from build123d import *

# Parameters (mm, degrees)
EXTRUDE_1_DEPTH     = 95
CUT_EXTRUDE_1_REACH = 144.466
SKETCH_2_R          = 3


with BuildPart() as part:
    # 草图1 → 凸台-拉伸1 (new body)
    with BuildSketch(Plane.XY):
        Polygon((-43.550332336, 35.659057411), (-38.550332336, 35.659057411), (-38.550332336, -8.806832193), (56.449667664, -8.806832193), (56.449667664, -14.340942589), (-43.550332336, -14.340942589), align=None)
    extrude(amount=EXTRUDE_1_DEPTH)

    # 草图2 → 切除-拉伸1 (cut, up to next)
    with BuildSketch(Plane.ZY.offset(43.550332336), mode=Mode.PRIVATE) as cut_extrude_1_sk1:
        with Locations((27, 8.8)):
            Circle(SKETCH_2_R)
    cut_extrude_1_tool1 = extrude(cut_extrude_1_sk1.sketch, amount=-CUT_EXTRUDE_1_REACH, mode=Mode.PRIVATE) & part.part
    add(cut_extrude_1_tool1.solids().sort_by_distance((-43.550332, 8.8, 27))[0], mode=Mode.SUBTRACT)


solid = part.part
Geometry: final body of the model. Coordinates: model frame, mm. A direction names the side the tool comes from. Round coordinates to 2 decimals unless told otherwise and drop trailing zeros. Loops run counter-clockwise (first coordinate to the right, second up) from the corner with the lowest first, then second, coordinate; pieces in that order, holes last. Notation, with made-up numbers: M 23.5,-37.75 L 81.5,-37.75 A17 ccw 81.5,-20.75 Z; hole C 61,23 d7. An arc over 180 degrees is marked long. Put each result on its own line as item: value. Start each with the question number.
(1) Section query C-C (z = 57). Return loops of the section in (x, y), then the cut area to 3 significant figures.
(2) Material intervals for line 1 along Y through (x, z) = (-40, 27); line 2 along X through (y, z) = (10, 88); line 3 along Y through (x, z) = (16, 49.5), sorted ascending. Write a range as [from, to].
(3) Draft query along Z for faces 3 (the face through (-4, -10, 0)), 4 (the face through (-41.1, 8.9, 24)), 5 (the face through (8, -8.807, 47)). Return one class per face: +Z half, -Z half, draft (parallel to the pull), parting line (faces both ways), or undercut.
(4) Section query A-A (y = 8.8). Return loops of the section in (x, z).
(5) Contact query for flat-ended pins moving along their axis: pin 1 Ø3 at (y, z) = (24.5, 34) entering from +X; pin 2 Ø10 at (x, z) = (-33, 85) entering from +Y. Output: stop coordinate, or through.
(6) Set-up query: faces 1 (the face through (56.45, -12, 47)), 2 (the face through (-38.55, 14, 47)). Return all of +Z, -Z, +X, -X, +Y, -Y with unobstructed straight access to the full face (end or side cutting, diameter ignored); none if empty.
(7) Section query D-D (y = 18). Return loops of the section in (x, z).
(8) Section query B-B (z = 27). Return loops of the section in (x, y), then the cut area to 3 significant figures.
Findings below:
1. outline: M -43.55,-14.34 L 56.45,-14.34 L 56.45,-8.81 L -38.55,-8.81 L -38.55,35.66 L -43.55,35.66 Z
1. area: 776 mm2
2. line 1: y = [-14.34, 5.8], [11.8, 35.66]
2. line 2: x = [-43.55, -38.55]
2. line 3: y = [-14.34, -8.81]
3. face 3: -Z half
3. face 4: undercut
3. face 5: draft
4. outline: M -43.55,0 L -38.55,0 L -38.55,24 L -43.55,24 Z; M -43.55,30 L -38.55,30 L -38.55,95 L -43.55,95 Z
5. pin 1: stops at x = -38.55
5. pin 2: stops at y = -8.81
6. face 1: +Z, -Z, +X, +Y, -Y
6. face 2: +Z, -Z, +X, +Y
7. outline: M -43.55,0 L -38.55,0 L -38.55,95 L -43.55,95 Z
8. outline: M -43.55,-14.34 L 56.45,-14.34 L 56.45,-8.81 L -38.55,-8.81 L -38.55,5.8 L -43.55,5.8 Z; M -43.55,11.8 L -38.55,11.8 L -38.55,35.66 L -43.55,35.66 Z
8. area: 746 mm2
